```python
from build123d import *

# Parameters (mm, degrees)
CYLINDER031_R     = 1.6
CYLINDER031_DEPTH = 28
BOX041_W          = 8
BOX041_H          = 10.5
BOX041_DEPTH      = 2.5
CYLINDER013_R     = 1.1
CYLINDER013_DEPTH = 28
CYLINDER012_R     = 1.1
CYLINDER012_DEPTH = 28
CYLINDER011_R     = 1.6
CYLINDER011_DEPTH = 28
CYLINDER010_R     = 3
CYLINDER010_DEPTH = 4
BOX037_W          = 8
BOX037_H          = 10.5
BOX037_DEPTH      = 10
BOX017_W          = 4
BOX017_H          = 52
BOX017_DEPTH      = 1.5
BOX016_W          = 77
BOX016_H          = 48
BOX016_DEPTH      = 40
FILLET009_R       = 8
BOX015_W          = 8
BOX015_H          = 52
BOX015_DEPTH      = 26
FILLET008_R       = 9
BOX039_W          = 15
BOX039_H          = 10.5
BOX039_DEPTH      = 7
BOX038_W          = 8
BOX038_H          = 10.5
BOX038_DEPTH      = 10
FILLET011_R       = 5


with BuildPart() as cylinder031:
    # Cylinder031 → Cylinder031 (new body)
    with BuildSketch(Plane(origin=(74, 76, -28), x_dir=(1, 0, 0), z_dir=(0, 0, 1))):
        Circle(CYLINDER031_R)
    extrude(amount=CYLINDER031_DEPTH)


with BuildPart() as cut031:
    # Box041 → Box041 (new body)
    with BuildSketch(Plane(origin=(70, 71.5, -26), x_dir=(1, 0, 0), z_dir=(0, 0, 1))):
        with Locations((4, 5.25)):
            Rectangle(BOX041_W, BOX041_H)
    extrude(amount=BOX041_DEPTH)

    # Cut031: cut Cylinder031
    add(cylinder031.part, mode=Mode.SUBTRACT)


with BuildPart() as cut031_1:
    # Cut031 placement: moved
    add(cut031.part.moved(Location((40, 0, 26))))


with BuildPart() as cylinder013:
    # Cylinder013 → Cylinder013 (new body)
    with BuildSketch(Plane(origin=(74, 118, -26), x_dir=(1, 0, 0), z_dir=(0, 0, 1))):
        Circle(CYLINDER013_R)
    extrude(amount=CYLINDER013_DEPTH)


with BuildPart() as fusion009:
    # Cylinder012 → Cylinder012 (new body)
    with BuildSketch(Plane(origin=(74, 94, -26), x_dir=(1, 0, 0), z_dir=(0, 0, 1))):
        Circle(CYLINDER012_R)
    extrude(amount=CYLINDER012_DEPTH)

    # Fusion009: union Cylinder013
    add(cylinder013.part)


with BuildPart() as fusion009_1:
    # Fusion009 placement: moved
    add(fusion009.part.moved(Location((54, 0, 0))))


with BuildPart() as cylinder011:
    # Cylinder011 → Cylinder011 (new body)
    with BuildSketch(Plane(origin=(74, 79, -26), x_dir=(1, 0, 0), z_dir=(0, 0, 1))):
        Circle(CYLINDER011_R)
    extrude(amount=CYLINDER011_DEPTH)


with BuildPart() as fusion008:
    # Cylinder010 → Cylinder010 (new body)
    with BuildSketch(Plane(origin=(74, 79, -26), x_dir=(1, 0, 0), z_dir=(0, 0, 1))):
        Circle(CYLINDER010_R)
    extrude(amount=CYLINDER010_DEPTH)

    # Fusion008: union Cylinder011
    add(cylinder011.part)


with BuildPart() as fusion008_1:
    # Fusion008 placement: moved
    add(fusion008.part.moved(Location((40, -3, 8))))


with BuildPart() as cube001:
    # Box037 → Box037 (new body)
    with BuildSketch(Plane(origin=(124, 71.5, -10), x_dir=(1, 0, 0), z_dir=(0, 0, 1))):
        with Locations((4, 5.25)):
            Rectangle(BOX037_W, BOX037_H)
    extrude(amount=BOX037_DEPTH)


with BuildPart() as box017:
    # Box017 → Box017 (new body)
    with BuildSketch(Plane(origin=(72, 71.5, -26), x_dir=(1, 0, 0), z_dir=(0, 0, 1))):
        with Locations((2, 26)):
            Rectangle(BOX017_W, BOX017_H)
    extrude(amount=BOX017_DEPTH)


with BuildPart() as fillet009:
    # Box016 → Box016 (new body)
    with BuildSketch(Plane(origin=(62, 82, -27), x_dir=(1, 0, 0), z_dir=(0, 0, 1))):
        with Locations((38.5, 24)):
            Rectangle(BOX016_W, BOX016_H)
    extrude(amount=BOX016_DEPTH)

    # Fillet009
    fillet009_edges = [fillet009.edges().sort_by_distance(p)[0] for p in [
        (100.5, 82, -27),
        (100.5, 82, 13),
        (100.5, 130, -27),
        (100.5, 130, 13),
    ]]
    fillet(fillet009_edges, radius=FILLET009_R)


with BuildPart() as fillet009_1:
    # Fillet009 placement: moved
    add(fillet009.part.moved(Location((0, 0, 4))))


with BuildPart() as cut027:
    # Box015 → Box015 (new body)
    with BuildSketch(Plane(origin=(70, 71.5, -26), x_dir=(1, 0, 0), z_dir=(0, 0, 1))):
        with Locations((4, 26)):
            Rectangle(BOX015_W, BOX015_H)
    extrude(amount=BOX015_DEPTH)

    # Cut012: cut Fillet009
    add(fillet009_1.part, mode=Mode.SUBTRACT)

    # Fillet008
    fillet008_edges = [cut027.edges().sort_by_distance(p)[0] for p in [
        (74, 71.5, -26),
    ]]
    fillet(fillet008_edges, radius=FILLET008_R)

    # Cut011: cut Box017
    add(box017.part, mode=Mode.SUBTRACT)


with BuildPart() as cut027_1:
    # Cut011 placement: moved
    add(cut027.part.moved(Location((54, 0, 0))))

    # Cut027: cut Cube001
    add(cube001.part, mode=Mode.SUBTRACT)


with BuildPart() as cube003:
    # Box039 → Box039 (new body)
    with BuildSketch(Plane(origin=(110, 71.5, -17), x_dir=(1, 0, 0), z_dir=(0, 0, 1))):
        with Locations((7.5, 5.25)):
            Rectangle(BOX039_W, BOX039_H)
    extrude(amount=BOX039_DEPTH)


with BuildPart() as fusion035:
    # Box038 → Box038 (new body)
    with BuildSketch(Plane(origin=(110, 71.5, -10), x_dir=(1, 0, 0), z_dir=(0, 0, 1))):
        with Locations((4, 5.25)):
            Rectangle(BOX038_W, BOX038_H)
    extrude(amount=BOX038_DEPTH)

    # Fusion033: union Cut027, Cube003
    add(cut027_1.part)
    add(cube003.part)

    # Fillet011
    fillet011_edges = [fusion035.edges().sort_by_distance(p)[0] for p in [
        (110, 76.75, -17),
    ]]
    fillet(fillet011_edges, radius=FILLET011_R)

    # Cut028: cut Fusion008
    add(fusion008_1.part, mode=Mode.SUBTRACT)

    # Cut029: cut Fusion009
    add(fusion009_1.part, mode=Mode.SUBTRACT)

    # Fusion035: union Cut031
    add(cut031_1.part)


solid = fusion035.part
```
Here's how the part is built. I have some questions about the finished solid (model axes, mm). A direction names the side the tool comes from. Coordinates: 2 decimals unless noted, no trailing zeros. Order: outer loops, then holes, each group sorted by start corner. A loop starts at its lowest first (then second) coordinate and runs counter-clockwise, first axis right, second up.
Item 1: If we section it at B-B, the plane y = 118: List the corners of the cut face in (x, z) for me, then the cut area to 3 significant figures.
Response values:
outline: (124, -26) - (126, -26) - (126, -24.5) - (126.9, -24.5) - (126.9, -23) - (124, -23) - close; (129.1, -24.5) - (130, -24.5) - (130, -26) - (132, -26) - (132, -23) - (129.1, -23) - close
area: 14.7 mm2
Item 2: If we section it at D-D, the plane x = 114: List the corners of the cut face in (y, z) for me.
Response values:
outline: (71.5, -16.9) - (73, -16.9) - (73, -14) - (74.4, -14) - (74.4, 2.5) - (71.5, 2.5) - close; (77.6, -14) - (79, -14) - (79, -16.9) - (82, -16.9) - (82, 2.5) - (77.6, 2.5) - close
Item 3: I need wall thicknesses on probe 1 along X at (y, z) = (76, -7.75); probe 2 along Y at (x, z) = (128, -23.95); probe 3 along Y at (x, z) = (128, -23.3). Which ranges of each line are inside material? Lowest first, please.
Response values:
probe 1: x = 110 to 112.4, 115.6 to 118
probe 2: y = 74.78 to 92.9, 95.1 to 116.9, 119.1 to 123.5
probe 3: y = 74.07 to 92.9, 95.1 to 116.9, 119.1 to 123.5
Item 4: If we section it at A-A, the plane x = 128: List the corners of the cut face in (y, z) for me.
Response values:
outline: (71.5, -17) arc R9 ccw to (75.53, -24.5) - (92.9, -24.5) - (92.9, -23) - (90, -23) arc R8 cw to (82, -15) - (82, -10) - (71.5, -10) - close; (95.1, -24.5) - (116.9, -24.5) - (116.9, -23) - (95.1, -23) - close; (119.1, -24.5) - (123.5, -24.5) - (123.5, -22.86) arc R8 cw to (122, -23) - (119.1, -23) - close
Item 5: If we section it at C-C, the plane z = -4.5: List the corners of the cut face in (x, y) for me.
Response values:
outline: (110, 71.5) - (118, 71.5) - (118, 82) - (110, 82) - close; hole circle Ø3.2 at (114, 76)
Item 6: I'm going to push flat-ended pins straight in: pin 1 Ø4 at (x, z) = (128.5, -12.5) entering from +Y; pin 2 Ø3 at (x, y) = (114, 77) entering from -Z; pin 3 Ø6 at (y, z) = (90.5, -22.5) entering from -X. Where does each tip first touch, or does it pass through?
Response values:
pin 1: stops at y = 82
pin 2: stops at z = -14
pin 3: stops at x = 124
Item 7: Thinking about a two-plate mould opening in X: for faces 5 (the face through (132, 91.4, -23.4)), 6 (the face through (116.86, 76.9, -15.19)), 7 (the face through (126, 99, -25)), 8 (the face through (125, 102, -26)), which applies, pulls with the +X half, pulls with the -X half, needs draft (parallel to the pull), parting line crosses it, or undercut?
Response values:
face 5: pulls with the +X half
face 6: undercut
face 7: undercut
face 8: needs draft
Item 8: Which directions (+Z, -Z, +X, -X, +Y, -Y) give clear straight access to the entire face, cutting with the end or side of a thin tool? Please do faces 1 (the face through (119, 77, -17)), 2 (the face through (125, 77, -10)), 3 (the face through (116, 82, -10)), 4 (the face through (130, 99, -25)).
Response values:
face 1: -Z, -X, +Y, -Y
face 2: +Z, +X, +Y, -Y
face 3: +Z, -X, +Y
face 4: -Z, +Y, -Y
